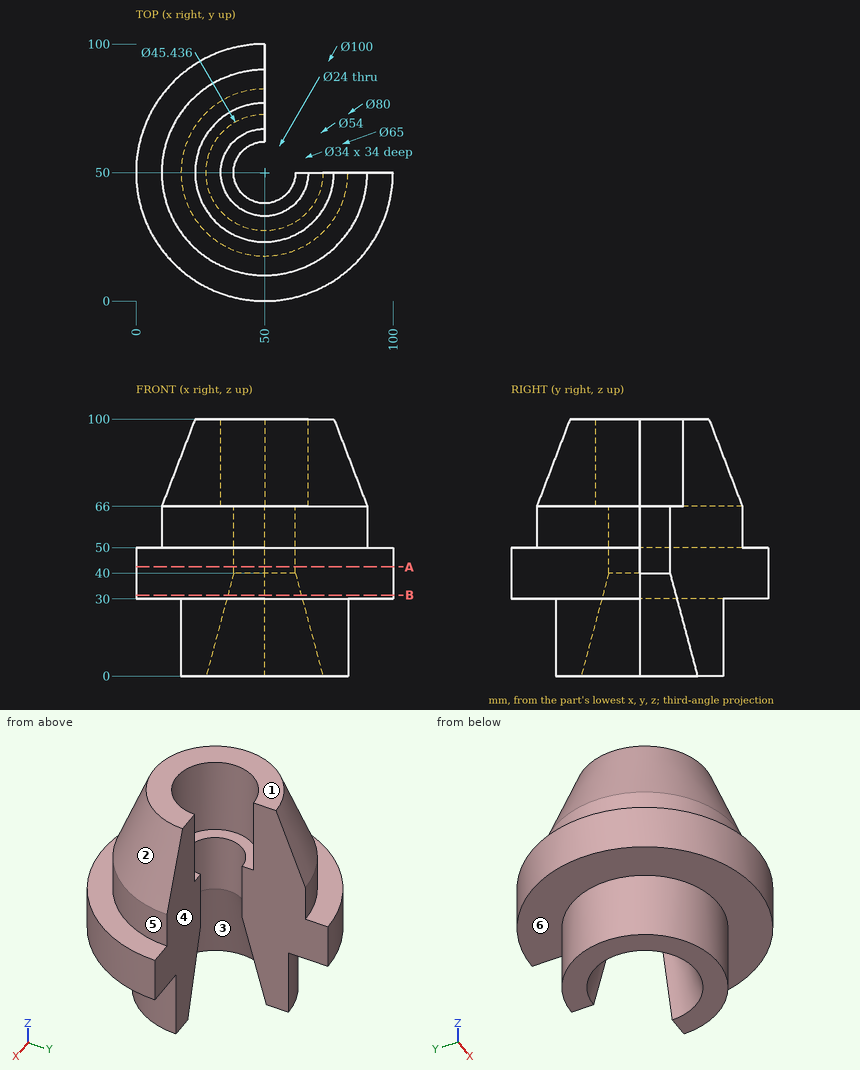
The figure shows three views and two pictorial views of one solid part (mm, origin at its lowest corner). Answer the questions. A direction names the side the tool comes from. Round coordinates to 2 decimals unless told otherwise and drop trailing zeros. Loops run counter-clockwise (first coordinate to the right, second up) from the corner with the lowest first, then second, coordinate; pieces in that order, holes last. Notation, with made-up numbers: (-25.5, -10.5) - (5.5, -10.5) arc R11 ccw to (5.5, 2.5) - close; hole circle Ø9 at (62.5, -14.5). An arc over 180 degrees is marked (long way). Use one line per item in the form item = value. Start each with the question number.
(1) Which of the six approach directions +Z, -Z, +X, -X, +Y, -Y give full straight-line access (tool end or side, diameter ignored) to the marked faces 4, 5 and 6?
(2) Consider line 1 (Z direction, x = 7, y = 68.5); line 2 (X direction, y = 36, z = 73); line 3 (Y direction, x = 49, z = 94). Determine where each line is inside the solid, lowest interval first.
(3) Find section A-A on z = 42.5. Determine the outline of the cut face in (x, y).
(4) Flat-ended cylindrical pins translate along their axes: P1, Ø1, axis at y = 20.5, z = 14.5, coming from the +X side; P2, Ø4, axis at y = 37, z = 11.5, coming from the +X side; P3, Ø2, axis at x = 40.5, z = 20, coming from the -Y side; P4, Ø1, axis at x = 52, y = 65, coming from the +Z side. Find the tip coordinate at first contact, or state that the pin passes through.
(5) Find section B-B on z = 31.5. Determine the outline of the cut face in (x, y) (1 decimal), and give its area (3 significant figures).
(6) Determine the mould class of the marked faces 1, 2 and 3 for opening direction X: +X half, -X half, draft (parallel to the pull), parting line (faces both ways), or undercut.
Answer list:
q1.face_4 = +Z, -Z, +X, +Y
q1.face_5 = +Z
q1.face_6 = -Z
q2.line_1 = 30 to 50
q2.line_2 = 15.4 to 40.36, 59.64 to 84.6
q2.line_3 = 20.72 to 33.03, 66.97 to 79.28
q3.outline = (50, 62) - (50, 100) arc R50 ccw (long way) to (100, 50) - (62, 50) arc R12 cw (long way) to start
q4.P1 = 64.67
q4.P2 = 80.58
q4.P3 = 18.63
q4.P4 = through
q5.outline = (50, 64.3) - (50, 100) arc R50 ccw (long way) to (100, 50) - (64.3, 50) arc R14.3 cw (long way) to start
q5.area = 5,410 mm^2
q6.face_1 = draft
q6.face_2 = parting line
q6.face_3 = undercut
